The model under review builds one solid part; all positions refer to its coordinate system, in mm. A direction names the side the tool comes from. Round coordinates to 2 decimals unless told otherwise and drop trailing zeros. Order: outer loops, then holes, each group sorted by start corner. A loop starts at its lowest first (then second) coordinate and runs counter-clockwise, first axis right, second up. Notation, with made-up numbers: M 79.5,-16 L 134.5,-16 A19 ccw 134.5,2 Z; hole C -26.75,79.25 d6. An arc over 180 degrees is marked long. Use a Markdown table: item, result. Add a question column.
1. Consider section C-C on z = -2.5. State the section outline as (x, y) points, then the cut area to 3 significant figures.
2. Consider section A-A on z = 5. State the section outline as (x, y) points, then the cut area to 3 significant figures.
3. The part is to be moulded in two halves that separate along X. For faces 5 (the flat face through (0, 2, 6)), 6 (the flat face through (-7.5, 0, 0.5)), 7 (the flat face through (0, -1.5, 8)), say which applies: +X half, -X half, draft (parallel to the pull), parting line (faces both ways), or undercut.
4. To check wall thickness, follow probe 1 along X at (y, z) = (-1.1, 7.25); probe 2 along Y at (x, z) = (0, -3.95). State the ranges of each line that lie inside material, in increasing order.
5. For faces 1 (the flat face through (2, 0, 8)), 2 (the flat face through (-1.5, 0, 8)), 3 (the flat face through (-5, 0, 1)), 4 (the flat face through (0.2, 0, -4)), list the 3-axis set-ups (+Z, -Z, +X, -X, +Y, -Y) from which the entire face can be reached by the end or side of a thin tool; tool diameter is ignored.
6. Insertion check: P1, Ø1.2, axis at x = -2.5, y = 0, coming from the -Z side; P2, Ø1.5, axis at y = -1, z = 9, coming from the -X side; P3, Ø2, axis at y = 0, z = 9, coming from the +X side; P4, Ø4, axis at x = 4.5, z = 13, coming from the +Y side. Each pin has a flat end and moves straight along its axis. Give the tip position at first contact, or say it passes through.
7. Consider section B-B on y = 0. State the section outline as (x, z) points, then the cut area to 4 significant figures.
from build123d import *

# Parameters (mm, degrees)
SKETCH_8_W      = 4
SKETCH_8_H      = 4
EXTRUDE_5_DEPTH = 16
SHELL_2_T       = -0.5
SKETCH_9_R      = 1
EXTRUDE_6_DEPTH = 4
SKETCH_10_R     = 1
SKETCH_10_R_2   = 0.849026748
EXTRUDE_7_DEPTH = 0.05
SKETCH_11_W     = 5.5
SKETCH_11_H     = 4
EXTRUDE_8_DEPTH = 1


with BuildPart() as part:
    # Эскиз8 → Бобышка-Вытянуть5 (new body)
    with BuildSketch(Plane.XY):
        Rectangle(SKETCH_8_W, SKETCH_8_H)
    extrude(amount=EXTRUDE_5_DEPTH)

    # Оболочка2
    shell_2_openings = [part.faces().sort_by_distance(p)[0] for p in [
        (0, 0, 16),
    ]]
    offset(amount=SHELL_2_T, openings=shell_2_openings, kind=Kind.INTERSECTION)

    # Эскиз9 → Бобышка-Вытянуть6 (add)
    with BuildSketch(Plane(origin=(0, 0, 0), x_dir=(-1, 0, 0), z_dir=(0, 0, -1))):
        Circle(SKETCH_9_R)
    extrude(amount=EXTRUDE_6_DEPTH)

    # Эскиз10 → Бобышка-Вытянуть7 (add)
    # profile 1 of 2: a face of its own
    with BuildSketch(Plane(origin=(0, 0, -4), x_dir=(-1, 0, 0), z_dir=(0, 0, -1))):
        Circle(SKETCH_10_R)
        Circle(SKETCH_10_R_2, mode=Mode.SUBTRACT)
    # profile 2 of 2: a face of its own
    with BuildSketch(Plane(origin=(0, 0, -4), x_dir=(-1, 0, 0), z_dir=(0, 0, -1))):
        with BuildLine():
            ThreePointArc((0, 0.556564641), (0.047474291, 0.655228966), (0.15419684, 0.679698432))
            ThreePointArc((0.15419684, 0.679698432), (0.6969696, 0), (0.15419684, -0.679698432))
            ThreePointArc((0.15419684, -0.679698432), (0.047474291, -0.655228966), (0, -0.556564641))
            Line((0, -0.556564641), (0, 0.556564641))
        make_face()
    extrude(amount=EXTRUDE_7_DEPTH)

    # Эскиз11 → Бобышка-Вытянуть8 (add)
    with BuildSketch(Plane(origin=(0, 0, 0), x_dir=(-1, 0, 0), z_dir=(0, 0, -1))):
        with Locations((-4.75, 0)):
            Rectangle(SKETCH_11_W, SKETCH_11_H)
        with Locations((4.75, 0)):
            Rectangle(SKETCH_11_W, SKETCH_11_H)
    extrude(amount=-EXTRUDE_8_DEPTH)


solid = part.part
Answer block:
| question | item | result |
|---|---|---|
| 1 | outline | C 0,0 d2 |
| 1 | area | 3.14 mm^2 |
| 2 | outline | M -2,-2 L 2,-2 L 2,2 L -2,2 Z; hole M -1.5,-1.5 L 1.5,-1.5 L 1.5,1.5 L -1.5,1.5 Z |
| 2 | area | 7.00 mm^2 |
| 3 | face 5 | draft |
| 3 | face 6 | -X half |
| 3 | face 7 | undercut |
| 4 | probe 1 | -2 to -1.5, 1.5 to 2 |
| 4 | probe 2 | -1 to 1 |
| 5 | face 1 | +Z, +X, +Y, -Y |
| 5 | face 2 | +Z |
| 5 | face 3 | +Z, -X, +Y, -Y |
| 5 | face 4 | -Z |
| 6 | P1 | z = 0 |
| 6 | P2 | x = -2 |
| 6 | P3 | x = 2 |
| 6 | P4 | through |
| 7 | outline | M -7.5,0 L -1,0 L -1,-4.05 L -0.85,-4.05 L -0.85,-4 L -0.7,-4 L -0.7,-4.05 L 0,-4.05 L 0,-4 L 0.85,-4 L 0.85,-4.05 L 1,-4.05 L 1,0 L 7.5,0 L 7.5,1 L 2,1 L 2,16 L 1.5,16 L 1.5,0.5 L -1.5,0.5 L -1.5,16 L -2,16 L -2,1 L -7.5,1 Z |
| 7 | area | 36.55 mm^2 |
